Part model, mm, in its own coordinate system. A direction names the side the tool comes from. Round coordinates to 2 decimals unless told otherwise and drop trailing zeros. Loops run counter-clockwise (first coordinate to the right, second up) from the corner with the lowest first, then second, coordinate; pieces in that order, holes last. Notation, with made-up numbers: (-18.75, 37) -> (7.25, 37) arc R9 ccw to (7.25, 52) -> close; hole circle Ø10 at (48.5, 86.25). An arc over 180 degrees is marked (long way). Use a Markdown table: item, result. Add a question column.
Item 1: Cut at A-A, the plane z = 0. List the corners of the cut face in (x, y), plus the area to 3 significant figures.
Item 2: Probe line 1 (X direction, y = 2, z = 0); line 2 (Z direction, x = 1, y = 8). List the from-to ranges inside material, lowest first. Write a range as [from, to].
Item 3: Which spindle directions (+Z, -Z, +X, -X, +Y, -Y) get a long thin tool onto all of the face, cutting with end or side? Do faces 5 (the face through (0, -1, 0)), 6 (the face through (0, 0, 0)). Say none if no direction does.
Item 4: Two-plate mould, pull along Z, no slides. Class faces 1 (the face through (0.9, 4.36, 2.86)), 2 (the face through (0, 4, 5.6)), 3 (the face through (-3, 9, 2)), 4 (the face through (0, 4, -5.6)): pulls with the +Z half, pulls with the -Z half, needs draft (parallel to the pull), parting line crosses it, or undercut.
Item 5: Cut at B-B, the plane x = 0. List the corners of the cut face in (y, z).
```python
from build123d import *

# Parameters (mm, degrees)
SKETCH2_W                                       = 11.2
SKETCH2_H                                       = 11.2
SKETCH2_R                                       = 3
BOSS_EXTRUDE1_DEPTH                             = 9
SKETCH3_W                                       = 11.2
SKETCH3_H                                       = 11.2
BOSS_EXTRUDE2_DEPTH                             = 1
FILLET1_SIZE                                    = 2
CSK_FOR_M3_FLAT_HEAD_MACHINE_SCREW1_D           = 3.4
CSK_FOR_M3_FLAT_HEAD_MACHINE_SCREW1_DEPTH       = 9
CSK_FOR_M3_FLAT_HEAD_MACHINE_SCREW1_CSINK_D     = 6.3
CSK_FOR_M3_FLAT_HEAD_MACHINE_SCREW1_CSINK_ANGLE = 90


with BuildPart() as part:
    # Sketch2 → Boss-Extrude1 (new body)
    with BuildSketch(Plane(origin=(0, 0, 0), x_dir=(1, 0, 0), z_dir=(0, 1, 0))):
        Rectangle(SKETCH2_W, SKETCH2_H)
        with Locations(Location((0, 0, 0), (0, 0, 270))):
            Circle(SKETCH2_R, mode=Mode.SUBTRACT)
    extrude(amount=BOSS_EXTRUDE1_DEPTH)

    # Sketch3 → Boss-Extrude2 (add)
    with BuildSketch(Plane.XZ):
        Rectangle(SKETCH3_W, SKETCH3_H)
    extrude(amount=BOSS_EXTRUDE2_DEPTH)

    # Fillet1
    # a fillet whose section is not a circle: 2 mm, written as the material it takes off along each edge
    with BuildSketch(Plane(origin=(5.6, -6, 5.6), x_dir=(-1, 0, 0), z_dir=(0, 1, 0)), Plane(origin=(-5.6, 14, 5.6), x_dir=(1, 0, 0), z_dir=(0, -1, 0))) as fillet1_piece_1:
        with BuildLine():
            add(Edge.make_bspline([(FILLET1_SIZE, 0), (FILLET1_SIZE * 0.831801948466, 0), (FILLET1_SIZE * 0.663603896932, 0), (FILLET1_SIZE * 0.292893218813, -FILLET1_SIZE * 0.0716919198361), (FILLET1_SIZE * 0.0716919198361, -FILLET1_SIZE * 0.292893218813), (0, -FILLET1_SIZE * 0.663603896932), (0, -FILLET1_SIZE * 0.831801948466), (0, -FILLET1_SIZE)], knots=[0, 0, 0, 0, 0, 0, 0.5, 0.5, 1, 1, 1, 1, 1, 1], degree=5))
            Line((0, -FILLET1_SIZE), (0, 0))
            Line((0, 0), (FILLET1_SIZE, 0))
        make_face()
    extrude(amount=20, mode=Mode.SUBTRACT)
    with BuildSketch(Plane(origin=(-5.6, 14, -5.6), x_dir=(1, 0, 0), z_dir=(0, -1, 0)), Plane(origin=(5.6, -6, -5.6), x_dir=(-1, 0, 0), z_dir=(0, 1, 0))) as fillet1_piece_2:
        with BuildLine():
            add(Edge.make_bspline([(FILLET1_SIZE, 0), (FILLET1_SIZE * 0.831801948466, 0), (FILLET1_SIZE * 0.663603896932, 0), (FILLET1_SIZE * 0.292893218813, FILLET1_SIZE * 0.0716919198361), (FILLET1_SIZE * 0.0716919198361, FILLET1_SIZE * 0.292893218813), (0, FILLET1_SIZE * 0.663603896932), (0, FILLET1_SIZE * 0.831801948466), (0, FILLET1_SIZE)], knots=[0, 0, 0, 0, 0, 0, 0.5, 0.5, 1, 1, 1, 1, 1, 1], degree=5))
            Line((0, FILLET1_SIZE), (0, 0))
            Line((0, 0), (FILLET1_SIZE, 0))
        make_face()
    extrude(amount=20, mode=Mode.SUBTRACT)

    # CSK for M3 Flat Head Machine Screw1
    with Locations(Plane(origin=(0, 9, 0), x_dir=(1, 0, 0), z_dir=(0, 1, 0))):
        with Locations((0, 0)):
            CounterSinkHole(CSK_FOR_M3_FLAT_HEAD_MACHINE_SCREW1_D / 2, CSK_FOR_M3_FLAT_HEAD_MACHINE_SCREW1_CSINK_D / 2, depth=CSK_FOR_M3_FLAT_HEAD_MACHINE_SCREW1_DEPTH, counter_sink_angle=CSK_FOR_M3_FLAT_HEAD_MACHINE_SCREW1_CSINK_ANGLE)


solid = part.part
```
A:
| question | item | result |
|---|---|---|
| 1 | outline | (-5.6, -1) -> (5.6, -1) -> (5.6, 9) -> (3.15, 9) -> (3, 8.85) -> (3, 0) -> (-3, 0) -> (-3, 8.85) -> (-3.15, 9) -> (-5.6, 9) -> close |
| 1 | area | 58.0 mm^2 |
| 2 | line 1 | x = [-5.6, -3], [3, 5.6] |
| 2 | line 2 | z = [-5.6, -2.83], [2.83, 5.6] |
| 3 | face 5 | +Z, -Z, +X, -X, -Y |
| 3 | face 6 | +Y |
| 4 | face 1 | undercut |
| 4 | face 2 | pulls with the +Z half |
| 4 | face 3 | needs draft |
| 4 | face 4 | pulls with the -Z half |
| 5 | outline | (-1, -5.6) -> (9, -5.6) -> (9, -3.15) -> (8.85, -3) -> (0, -3) -> (0, 3) -> (8.85, 3) -> (9, 3.15) -> (9, 5.6) -> (-1, 5.6) -> close |
